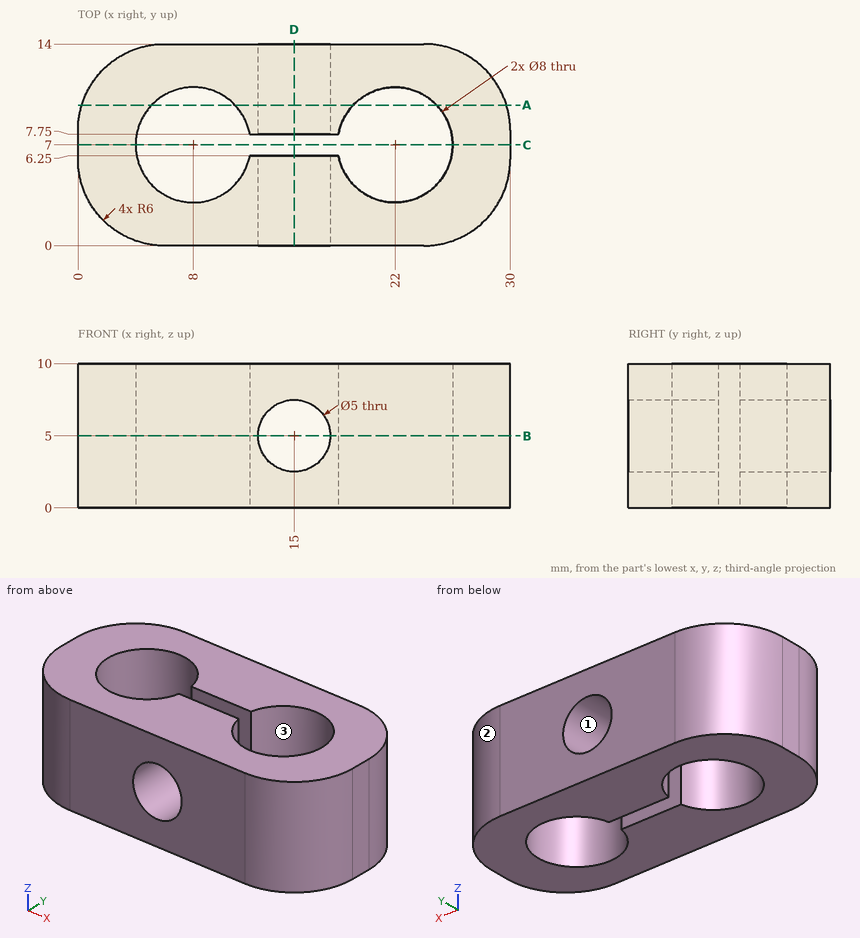
The figure shows three views and two pictorial views of one solid part (mm, origin at its lowest corner). Answer the questions. Round coordinates to 2 decimals unless told otherwise and drop trailing zeros. Loops run counter-clockwise (first coordinate to the right, second up) from the corner with the lowest first, then second, coordinate; pieces in that order, holes last. Notation, with made-up numbers: M -21,67 L -8,67 A25 cw -8,99 Z; hole C -38,15 d10. An arc over 180 degrees is marked long. Return JSON: item names as keys, results as strings.
Q1. Find section A-A, the plane y = 9.75. Determine the outline of the cut face in (x, z).
Results list:
{"outline": "M 0.26,0 L 5.1,0 L 5.1,10 L 0.26,10 Z; M 10.9,0 L 19.1,0 L 19.1,10 L 10.9,10 Z; M 24.9,0 L 29.74,0 L 29.74,10 L 24.9,10 Z; hole C 15,5 d5"}
Q2. Find section D-D, the plane x = 15. Determine the outline of the cut face in (y, z).
Results list:
{"outline": "M 0,0 L 6.25,0 L 6.25,2.5 L 0,2.5 Z; M 0,7.5 L 6.25,7.5 L 6.25,10 L 0,10 Z; M 7.75,0 L 14,0 L 14,2.5 L 7.75,2.5 Z; M 7.75,7.5 L 14,7.5 L 14,10 L 7.75,10 Z"}
Q3. Each of these flat-tipped pins is pushed along its axis until it touches: pin 1 Ø8 at (x, y) = (6, 4.5) entering from -Z; pin 2 Ø2 at (y, z) = (2, 2.5) entering from -X. Where does it stop, or does it pass through?
Results list:
{"pin 1": "stops at z = 0", "pin 2": "stops at x = 0.8"}
Q4. Find section C-C, the plane y = 7. Determine the outline of the cut face in (x, z).
Results list:
{"outline": "M 0,0 L 4,0 L 4,10 L 0,10 Z; M 26,0 L 30,0 L 30,10 L 26,10 Z"}
Q5. Find section B-B, the plane z = 5. Determine the outline of the cut face in (x, y), plus the area to 3 significant figures.
Results list:
{"outline": "M 0,6 A6 ccw 6,0 L 12.5,0 L 12.5,6.25 L 11.93,6.25 A4 cw long 11.93,7.75 L 12.5,7.75 L 12.5,14 L 6,14 A6 ccw 0,8 Z; M 17.5,0 L 24,0 A6 ccw 30,6 L 30,8 A6 ccw 24,14 L 17.5,14 L 17.5,7.75 L 18.07,7.75 A4 cw long 18.07,6.25 L 17.5,6.25 Z", "area": "217 mm2"}
Q6. The mould has two halves that part along Y. Classify the marked faces 1, 2 and 3: released by +Y, released by -Y, zero draft, split by the parting line, or undercut.
Results list:
{"face 1": "zero draft", "face 2": "released by +Y", "face 3": "undercut"}
Q7. Find the intervals of material crossed by line 1 along Y through (x, z) = (8, 7); line 2 along X through (y, z) = (7, 7.75); line 3 along Z through (x, y) = (15, 10.5), in increasing order. Write a range as from..to.
Results list:
{"line 1": "y = 0..3, 11..14", "line 2": "x = 0..4, 26..30", "line 3": "z = 0..2.5, 7.5..10"}
